Autodesk Inventor part; units mm, degrees
ref_plane "YZ Plane" through (0, 0, 0) normal (1, 0, 0) x (0, 1, 0)
ref_plane "XZ Plane" through (0, 0, 0) normal (0, 1, 0) x (-1, 0, 0)
ref_plane "XY Plane" through (0, 0, 0) normal (0, 0, 1) x (1, 0, 0)
sketch "Sketch1" plane through (0, 0, 0) normal (0, 0, 1) x (1, 0, 0)
  line L0 (2.8868, 0) -> (1.4434, -2.5)
  line L1 (1.4434, -2.5) -> (-1.4434, -2.5)
  line L2 (-1.4434, -2.5) -> (-2.8868, 0)
  line L3 (-2.8868, 0) -> (-1.4434, 2.5)
  line L4 (-1.4434, 2.5) -> (1.4434, 2.5)
  line L5 (1.4434, 2.5) -> (2.8868, 0)
  point P0 (0, 0)
  point P1 (0, 0)
  dimension "d0" = 5
extrude "Extrusion1" add sketch "Sketch1" along normal blind 5
sketch "Sketch2" plane through (0, 0, 5) normal (0, 0, 1) x (1, 0, 0)
  circle A0 centre (0, 0) radius 1.5
  dimension "d3" = 3
extrude "Extrusion2" add sketch "Sketch2" along normal blind 6
sketch "Sketch3" plane through (0, 0, 0) normal (0, 0, -1) x (-1, 0, 0)
  circle A0 centre (0, 0) radius 1.5
  dimension "d6" = 3
extrude "Extrusion3" cut sketch "Sketch3" against normal blind 4
sketch "Sketch4" plane through (0, 0, 4) normal (0, 0, -1) x (-1, 0, 0)
  circle A0 centre (0, 0) radius 1.5
extrude "Extrusion4" cut sketch "Sketch4" against normal through all
properties part number "Spacer5mm_m3_970050351"
Geometry check sheet. Reference: the model listing, model coordinates, mm. Coordinates: 2 decimals unless noted, no trailing zeros. Order: outer loops, then holes, each group sorted by start corner. A loop starts at its lowest first (then second) coordinate and runs counter-clockwise, first axis right, second up. Notation, with made-up numbers: (12.5, 44) - (61.5, 44) arc R20 cw to (61.5, 63) - close; hole circle Ø11 at (0, -33). An arc over 180 degrees is marked (long way). Answer in a Markdown table with one row per item. Add a question column.
1) Material ranges on line 1 along Y through (x, z) = (0, 3.15); line 2 along Y through (x, z) = (-1.2, 2.65); line 3 along X through (y, z) = (-1.15, 2.2), recorded low to high. Write a range as [from, to].
2) Cross-section at C-C, the plane z = 0.35. Record the cut outline in (x, y).
3) Cross-section at A-A, the plane x = 0. Record the cut outline in (y, z).
4) Cross-section at D-D, the plane y = -2.15. Record the cut outline in (x, z).
5) Release check for a two-part mould opening along Y. For faces 1 (the flat face through (1.24, 1.15, 5)), 2 (the flat face through (2.155, 1.267, 2.465)), 3 (the cylindrical face through (1.5, 0.07, 2.46)), 4 (the flat face through (2.175, -1.233, 2.465)) record: +Y half, -Y half, draft (parallel to the pull), parting line (faces both ways), or undercut.
6) Gauge pin test, flat ends, axial feed: P1, Ø1, axis at y = 1.5, z = 3, coming from the -X side; P2, Ø2, axis at x = -1.5, z = 2, coming from the -Y side; P3, Ø2, axis at y = 0.5, z = 1.5, coming from the +X side. Record the tip position at first contact, or that the pin passes through.
7) Cross-section at B-B, the plane y = -1.1. Record the cut outline in (x, z), then the cut area to 3 significant figures.
Check result:
| question | item | result |
|---|---|---|
| 1 | line 1 | y = [-2.5, -1.5], [1.5, 2.5] |
| 1 | line 2 | y = [-2.5, -0.9], [0.9, 2.5] |
| 1 | line 3 | x = [-2.22, -0.96], [0.96, 2.22] |
| 2 | outline | (-2.89, 0) - (-1.44, -2.5) - (1.44, -2.5) - (2.89, 0) - (1.44, 2.5) - (-1.44, 2.5) - close; hole circle Ø3 at (0, 0) |
| 3 | outline | (-2.5, 0) - (-1.5, 0) - (-1.5, 5) - (-2.5, 5) - close; (1.5, 0) - (2.5, 0) - (2.5, 5) - (1.5, 5) - close |
| 4 | outline | (-1.65, 0) - (1.65, 0) - (1.65, 5) - (-1.65, 5) - close |
| 5 | face 1 | draft |
| 5 | face 2 | +Y half |
| 5 | face 3 | undercut |
| 5 | face 4 | -Y half |
| 6 | P1 | stops at x = -2.31 |
| 6 | P2 | stops at y = -2.5 |
| 6 | P3 | stops at x = 2.89 |
| 7 | outline | (-2.25, 0) - (-1.02, 0) - (-1.02, 5) - (-2.25, 5) - close; (1.02, 0) - (2.25, 0) - (2.25, 5) - (1.02, 5) - close |
| 7 | area | 12.3 mm² |
